Input: part model. Units: mm. Frame: model coordinates. A direction names the side the tool comes from. Give positions to 0.01 mm unless a question says otherwise; leave off trailing zeros. Loops run counter-clockwise (first coordinate to the right, second up) from the corner with the lowest first, then second, coordinate; pieces in that order, holes last. Notation, with made-up numbers: (37.25, 60) -> (84.25, 60) arc R23 cw to (84.25, 83) -> close; hole circle Ø4 at (28, 2). An arc over 180 degrees is marked (long way). Answer as a JSON object with one key per item and string values.
```python
from build123d import *

# Parameters (mm, degrees)
BOSS_EXTRUDE1_DEPTH           = 12
CBORE_FOR_M6_SHCS1_AT_2_COUNT = 2
CBORE_FOR_M6_SHCS1_AT_2_PITCH = 50
CBORE_FOR_M6_SHCS1_AT_3_COUNT = 2
CBORE_FOR_M6_SHCS1_AT_3_PITCH = 90.138781887
CBORE_FOR_M6_SHCS1_AT_4_COUNT = 2
CBORE_FOR_M6_SHCS1_AT_4_PITCH = 75
CUT_EXTRUDE3_DEPTH            = 2
CBORE_FOR_M3_SHCS1_AT_2_COUNT = 2
CBORE_FOR_M3_SHCS1_AT_2_PITCH = 31
CBORE_FOR_M3_SHCS1_AT_3_COUNT = 2
CBORE_FOR_M3_SHCS1_AT_3_PITCH = 43.840620434
CBORE_FOR_M3_SHCS1_AT_4_COUNT = 2
CBORE_FOR_M3_SHCS1_AT_4_PITCH = 31
CHAMFER1_SIZE                 = 0.5
CHAMFER2_SIZE                 = 10


with BuildPart() as part:
    # Sketch1 → Boss-Extrude1 (new body)
    with BuildSketch(Plane(origin=(0, 0, 0), x_dir=(1, 0, 0), z_dir=(0, 1, 0))):
        Polygon((58, 41), (0, 41), (-42, 41), (-42, -41), (0, -41), (58, -41), align=None)
    extrude(amount=BOSS_EXTRUDE1_DEPTH)

    # Sketch14 → CBORE for M6 SHCS1 (revolve, cut)
    with BuildSketch(Plane(origin=(48.21, 12, -25), x_dir=(0, 0, 1), z_dir=(1, 0, 0))):
        Polygon((0, 0), (0, 12), (3.325, 12), (3.3, 11.975), (3.3, 6), (5.5, 6), (5.5, 0.025), (5.525, 0), align=None)
    cbore_for_m6_shcs1 = revolve(axis=Axis((48.21, 18.35, -25), (0, -1, 0)), mode=Mode.SUBTRACT)

    # CBORE for M6 SHCS1 at 2: CBORE for M6 SHCS1 ×2
    with Locations(*[(0, 0, i * CBORE_FOR_M6_SHCS1_AT_2_PITCH) for i in range(1, CBORE_FOR_M6_SHCS1_AT_2_COUNT)]):
        add(cbore_for_m6_shcs1, mode=Mode.SUBTRACT)

    # CBORE for M6 SHCS1 at 3: CBORE for M6 SHCS1 ×2
    with Locations(*[Vector(-0.8320502943378437, 0, 0.5547001962252291) * (i * CBORE_FOR_M6_SHCS1_AT_3_PITCH) for i in range(1, CBORE_FOR_M6_SHCS1_AT_3_COUNT)]):
        add(cbore_for_m6_shcs1, mode=Mode.SUBTRACT)

    # CBORE for M6 SHCS1 at 4: CBORE for M6 SHCS1 ×2
    with Locations(*[(-i * CBORE_FOR_M6_SHCS1_AT_4_PITCH, 0, 0) for i in range(1, CBORE_FOR_M6_SHCS1_AT_4_COUNT)]):
        add(cbore_for_m6_shcs1, mode=Mode.SUBTRACT)

    # Sketch9 → Cut-Extrude3 (cut)
    with BuildSketch(Plane(origin=(0, 12, 0), x_dir=(1, 0, 0), z_dir=(0, 1, 0))):
        Polygon((21.5, 19.5), (19.5, 21.5), (-19.5, 21.5), (-21.5, 19.5), (-21.5, -19.5), (-19.5, -21.5), (19.5, -21.5), (21.5, -19.5), align=None)
    extrude(amount=-CUT_EXTRUDE3_DEPTH, mode=Mode.SUBTRACT)

    # Sketch12 → CBORE for M3 SHCS1 (revolve, cut)
    with BuildSketch(Plane(origin=(-15.5, 0, -15.5), x_dir=(0, 0, -1), z_dir=(1, 0, 0))):
        Polygon((0, 0), (0, 10), (1.725, 10), (1.7, 9.975), (1.7, 3), (3.25, 3), (3.25, 0.025), (3.275, 0), align=None)
    cbore_for_m3_shcs1 = revolve(axis=Axis((-15.5, -6.35, -15.5), (0, 1, 0)), mode=Mode.SUBTRACT)

    # CBORE for M3 SHCS1 at 2: CBORE for M3 SHCS1 ×2
    with Locations(*[(i * CBORE_FOR_M3_SHCS1_AT_2_PITCH, 0, 0) for i in range(1, CBORE_FOR_M3_SHCS1_AT_2_COUNT)]):
        add(cbore_for_m3_shcs1, mode=Mode.SUBTRACT)

    # CBORE for M3 SHCS1 at 3: CBORE for M3 SHCS1 ×2
    with Locations(*[Vector(0.7071067811865476, 0, 0.7071067811865475) * (i * CBORE_FOR_M3_SHCS1_AT_3_PITCH) for i in range(1, CBORE_FOR_M3_SHCS1_AT_3_COUNT)]):
        add(cbore_for_m3_shcs1, mode=Mode.SUBTRACT)

    # CBORE for M3 SHCS1 at 4: CBORE for M3 SHCS1 ×2
    with Locations(*[(0, 0, i * CBORE_FOR_M3_SHCS1_AT_4_PITCH) for i in range(1, CBORE_FOR_M3_SHCS1_AT_4_COUNT)]):
        add(cbore_for_m3_shcs1, mode=Mode.SUBTRACT)

    # Chamfer1
    chamfer1_edges = [part.edges().sort_by_distance(p)[0] for p in [
        (0, 12, -21.5),
        (21.5, 12, 0),
        (-20.5, 12, -20.5),
        (-21.5, 12, 0),
        (-20.5, 12, 20.5),
        (0, 12, 21.5),
        (20.5, 12, 20.5),
        (20.5, 12, -20.5),
    ]]
    chamfer(chamfer1_edges, length=CHAMFER1_SIZE)

    # Chamfer2
    chamfer2_edges = [part.edges().sort_by_distance(p)[0] for p in [
        (-42, 6, 41),
        (-42, 6, -41),
    ]]
    chamfer(chamfer2_edges, length=CHAMFER2_SIZE)


solid = part.part
```
Q1. Draft query along Z for faces 4 (the flat face through (17, 3, -14)), 5 (the flat face through (-42, 6, 0)). Return one class per face: +Z half, -Z half, draft (parallel to the pull), parting line (faces both ways), or undercut.
Evaluation:
{"face 4": "undercut", "face 5": "draft"}
Q2. Section A-A, the plane x = 15.5. Give the number of separate pieces and of enclosed holes in the cut face, then the cut area to 3 significant figures.
Evaluation:
{"separate pieces": "3", "enclosed holes": "0", "area": "811 mm2"}
Q3. Section D-D, the plane z = 25. Return the cut outline in (x, y) (3 decimals).
Evaluation:
{"outline": "(-42, 0) -> (-30.115, 0) -> (-30.09, 0.025) -> (-30.09, 6) -> (-32.29, 6) -> (-32.29, 11.975) -> (-32.315, 12) -> (-42, 12) -> close; (-23.49, 0.025) -> (-23.465, 0) -> (44.885, 0) -> (44.91, 0.025) -> (44.91, 6) -> (42.71, 6) -> (42.71, 11.975) -> (42.685, 12) -> (-21.265, 12) -> (-21.29, 11.975) -> (-21.29, 6) -> (-23.49, 6) -> close; (51.51, 0.025) -> (51.535, 0) -> (58, 0) -> (58, 12) -> (53.735, 12) -> (53.71, 11.975) -> (53.71, 6) -> (51.51, 6) -> close"}
Q4. Pin query (flat end, axial travel): pin 1 (13 mm diameter, centred on x = -7.5, z = -1, fed in from +Y); pin 2 (3 mm diameter, centred on x = 16.5, z = -15.5, fed in from -Y). Return the tip coordinate at first contact, or that it passes through.
Evaluation:
{"pin 1": "stops at y = 10", "pin 2": "stops at y = 3"}
Q5. Access query for faces 1 (the flat face through (21, 11, -20)), 2 (the cylindrical face through (-25.53, 3.05, 28.05)), 3 (the flat face through (17, 3, 17)). Directions: +Z, -Z, +X, -X, +Y, -Y. A direction counts if a zero-diameter tool reaches every point of the face in a straight line with its end or side. Return the directions, or none.
Evaluation:
{"face 1": "+Y", "face 2": "+Y, -Y", "face 3": "-Y"}
Q6. Ray query, line 1 along Z through (x, y) = (48.21, 10.3); line 2 along X through (y, z) = (6.75, 15.5); line 3 along Z through (x, y) = (-15.5, 1.8). Return the intervals inside material, ascending.
Evaluation:
{"line 1": "z = -41 to -30.5, -19.5 to 19.5, 30.5 to 41", "line 2": "x = -42 to -17.2, -13.8 to 13.8, 17.2 to 58", "line 3": "z = -41 to -18.75, -12.25 to 12.25, 18.75 to 41"}
Q7. Section B-B, the plane z = -3.5. Return the cut outline in (x, y).
Evaluation:
{"outline": "(-42, 0) -> (58, 0) -> (58, 12) -> (22, 12) -> (21.5, 11.5) -> (21.5, 10) -> (-21.5, 10) -> (-21.5, 11.5) -> (-22, 12) -> (-42, 12) -> close"}
